For this review, use the dimensioned drawing (mm, ordinates from the lowest corner) and the shaded views. A direction names the side the tool comes from. Round coordinates to 2 decimals unless told otherwise and drop trailing zeros. Loops run counter-clockwise (first coordinate to the right, second up) from the corner with the lowest first, then second, coordinate; pieces in that order, holes last.
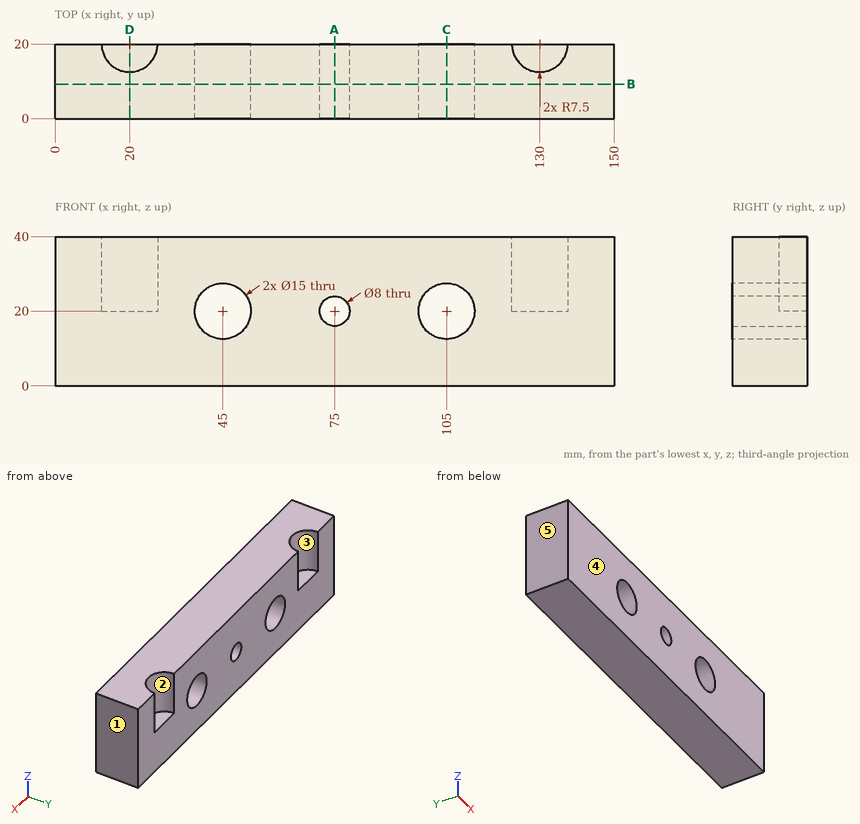
(1) Add section B-B (y = 9.25). Give the boundary of the cut face in (x, z).
(2) Add section C-C (x = 105). Give the boundary of the cut face in (y, z), plus the area to 3 significant figures.
(3) Add section D-D (x = 20). Give the boundary of the cut face in (y, z), plus the area to 3 significant figures.
(4) For the marked faces 1 and 2, list the 3-axis set-ups (+Z, -Z, +X, -X, +Y, -Y) from which the entire face can be reached by the end or side of a thin tool; tool diameter is ignored.
(5) Insertion check: pin 1 Ø9 at (x, z) = (75, 20) entering from +Y; pin 2 Ø4 at (x, y) = (131.5, 15.5) entering from +Z. Each pin has a flat end and moves straight along its axis. Give the tip position at first contact, or say it passes through.
(6) The part is to be moulded in two halves that separate along X. For the marked faces 3, 4 and 5, say which applies: pulls with the +X half, pulls with the -X half, needs draft (parallel to the pull), parting line crosses it, or undercut.
(7) Add section A-A (x = 75). Give the boundary of the cut face in (y, z), plus the area to 3 significant figures.
(8) For L1, parallel to X at y = 10.5, z = 20; L2, parallel to Z at x = 105, y = 10.25; L3, parallel to X at y = 14.75, z = 22.5, list the stretches that pass through material, from the lowest coordinate up.
Outcome:
1. outline: (0, 0) - (150, 0) - (150, 40) - (0, 40) - close; hole circle Ø15 at (45, 20); hole circle Ø8 at (75, 20); hole circle Ø15 at (105, 20)
2. outline: (0, 0) - (20, 0) - (20, 12.5) - (0, 12.5) - close; (0, 27.5) - (20, 27.5) - (20, 40) - (0, 40) - close
2. area: 500 mm2
3. outline: (0, 0) - (20, 0) - (20, 20) - (12.5, 20) - (12.5, 40) - (0, 40) - close
3. area: 650 mm2
4. face 1: +Z, -Z, +X, +Y, -Y
4. face 2: +Z, +Y
5. pin 1: stops at y = 20
5. pin 2: stops at z = 20
6. face 3: undercut
6. face 4: needs draft
6. face 5: pulls with the -X half
7. outline: (0, 0) - (20, 0) - (20, 16) - (0, 16) - close; (0, 24) - (20, 24) - (20, 40) - (0, 40) - close
7. area: 640 mm2
8. L1: x = 0 to 37.5, 52.5 to 71, 79 to 97.5, 112.5 to 150
8. L2: z = 0 to 12.5, 27.5 to 40
8. L3: x = 0 to 14.64, 25.36 to 37.93, 52.07 to 71.88, 78.12 to 97.93, 112.07 to 124.64, 135.36 to 150
